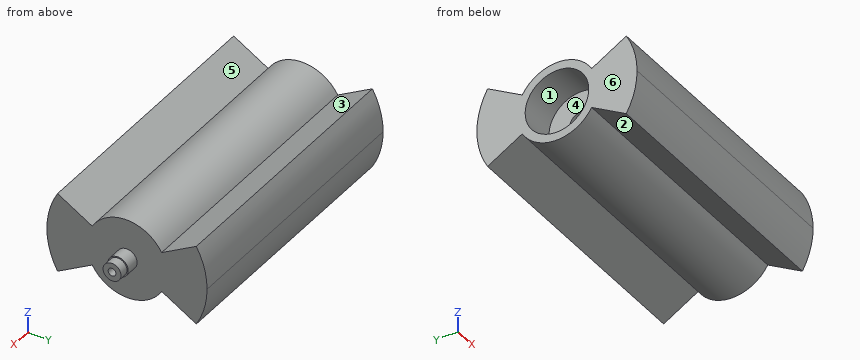
Autodesk Inventor part; units mm, degrees
ref_plane "YZ Plane" through (0, 0, 0) normal (1, 0, 0) x (0, 1, 0)
ref_plane "XZ Plane" through (0, 0, 0) normal (0, 1, 0) x (-1, 0, 0)
ref_plane "XY Plane" through (0, 0, 0) normal (0, 0, 1) x (1, 0, 0)
sketch "Sketch1" plane through (0, 0, 0) normal (1, 0, 0) x (0, 1, 0)
  circle A0 centre (0, 0) radius 17.5
  dimension "d1" = 35
extrude "Extrusion1" add sketch "Sketch1" along normal blind 118
sketch "Sketch2" plane through (0, 0, 0) normal (-1, 0, 0) x (0, 0, 1)
  circle A0 centre (0, 0) radius 13.9
  dimension "d4" = 27.8
extrude "Extrusion2" cut sketch "Sketch2" against normal blind 16
sketch "Sketch3" plane through (16, 0, 0) normal (-1, 0, 0) x (0, 0, 1)
  circle A0 centre (0, 0) radius 4.85
  dimension "d7" = 9.7
extrude "Extrusion3" cut sketch "Sketch3" against normal blind 4.2
sketch "Sketch4" plane through (20.2, 0, 0) normal (-1, 0, 0) x (0, 0, 1)
  circle A0 centre (0, 0) radius 1.7
  dimension "d10" = 3.4
extrude "Extrusion4" cut sketch "Sketch4" against normal blind 10
sketch "Sketch9" plane through (0, 0, 0) normal (1, 0, 0) x (0, 1, 0)
  circle A0 centre (0, 0) radius 1.7 construction
  circle A1 centre (0, 0) radius 35 construction
  line L0 (-35, 0) -> (-17.5, 0)
  circle A2 centre (0, 0) radius 17.5 construction
  line L1 (-15.1554, 8.75) -> (-30.3109, 17.5)
  arc A3 (-30.3109, 17.5) -> (-35, 0) centre (0, 0) ccw
  arc A4 (-15.1554, 8.75) -> (-17.5, 0) centre (0, 0) ccw
  dimension "d32" = 70
  dimension "d33" = 30
extrude "Extrusion8" add sketch "Sketch9" along normal up to surface (118 mm away)
sketch "Sketch10" plane through (118, 0, 0) normal (1, 0, 0) x (0, 0, -1)
  circle A0 centre (0, 0) radius 1.7
  circle A1 centre (0, 0) radius 3.925
  dimension "d36" = 7.85
extrude "Extrusion9" add sketch "Sketch10" along normal blind 10
sketch "Sketch12" plane through (118, 0, 0) normal (1, 0, 0) x (0, 0, -1)
  circle A0 centre (0, 0) radius 4.445
  dimension "d42" = 8.89
extrude "Extrusion11" add sketch "Sketch12" along normal blind 6
sketch "Sketch11" plane through (118, 0, 0) normal (1, 0, 0) x (0, 0, -1)
  circle A0 centre (0, 0) radius 4.85
  circle A1 centre (0, 0) radius 1.7
extrude "Extrusion10" cut sketch "Sketch11" against normal blind 20 from surface at 10 contours A1
mirror "Mirror1" about plane through (0, 0, 0) normal (0, 0, 1) of "Extrusion8"
mirror "Mirror2" about plane through (0, 0, 0) normal (0, 1, 0) of "Extrusion8", "Mirror1"
properties part number "newDrum_3DPrint"
Geometry check sheet. Reference: the model listing, model coordinates, mm. Face numbers are marked on the shaded views. A direction names the side the tool comes from. Round coordinates to 2 decimals unless told otherwise and drop trailing zeros. Write each loop counter-clockwise with the first axis right and the second up, starting at its lowest first coordinate (ties: lowest second). Pieces come first, ordered by that corner, then holes. Notation, with made-up numbers: (-29, -33.75) -> (-8, -33.75) arc R8 ccw to (-8, -29.75) -> close; hole circle Ø3 at (16, 28). An arc over 180 degrees is marked (long way). One line per item, written item: value. Start each with the question number.
(1) Access from +Z, -Z, +X, -X, +Y, -Y to the whole of each face (thin tool, end or side, straight path). Record for the marked faces 1, 2 and 3.
(2) Go/stop test with flat-tipped pins: pin 1 Ø1.5 at (x, z) = (49.5, -9) entering from +Y; pin 2 Ø1.7 at (y, z) = (-0.5, 0) entering from -X; pin 3 Ø8 at (y, z) = (-1, 5.5) entering from -X. Record where each tip stops, or that it passes through.
(3) Scan lines: line 1 (Y direction, x = 23.75, z = 0); line 2 (Y direction, x = 19, z = 0); line 3 (Y direction, x = 107, z = -16). Record each from-to range of solid material in increasing order. Write a range as [from, to].
(4) Cross-section at C-C, the plane x = 47. Record the cut outline in (y, z), and give its area (3 significant figures).
(5) Cross-section at B-B, the plane y = 0. Record the cut outline in (x, z) (3 decimals), and give its area (3 significant figures).
(6) Draft check along Z on the marked faces 4, 5 and 6. Enter one of: +Z half, -Z half, draft (parallel to the pull), parting line (faces both ways), or undercut.
(7) Cross-section at D-D, the plane z = -7. Record the cut outline in (x, y), and give its area (3 significant figures).
(8) Cross-section at A-A, the plane x = 13. Record the cut outline in (y, z), and give its area (3 significant figures).
Answer:
1. face 1: -X
1. face 2: -Z, +X, -X
1. face 3: +Z, +X, -X
2. pin 1: y = 34.01
2. pin 2: x = 30.2
2. pin 3: x = 16
3. line 1: [-35, -1.7], [1.7, 35]
3. line 2: [-35, -4.85], [4.85, 35]
3. line 3: [-31.13, -27.71], [-7.09, 7.09], [27.71, 31.13]
4. outline: (-35, 0) arc R35 ccw to (-30.31, -17.5) -> (-15.16, -8.75) arc R17.5 ccw to (15.16, -8.75) -> (30.31, -17.5) arc R35 ccw to (35, 0) arc R35 ccw to (30.31, 17.5) -> (15.16, 8.75) arc R17.5 ccw to (-15.16, 8.75) -> (-30.31, 17.5) arc R35 ccw to start
4. area: 1,920 mm²
5. outline: (0, -17.5) -> (118, -17.5) -> (118, -4.445) -> (124, -4.445) -> (124, -3.925) -> (128, -3.925) -> (128, -1.7) -> (108, -1.7) -> (108, 1.7) -> (128, 1.7) -> (128, 3.925) -> (124, 3.925) -> (124, 4.445) -> (118, 4.445) -> (118, 17.5) -> (0, 17.5) -> (0, 13.9) -> (16, 13.9) -> (16, 4.85) -> (20.2, 4.85) -> (20.2, 1.7) -> (30.2, 1.7) -> (30.2, -1.7) -> (20.2, -1.7) -> (20.2, -4.85) -> (16, -4.85) -> (16, -13.9) -> (0, -13.9) -> close
5. area: 3,630 mm²
6. face 4: undercut
6. face 5: +Z half
6. face 6: draft
7. outline: (0, -34.29) -> (118, -34.29) -> (118, 34.29) -> (0, 34.29) -> (0, 12.01) -> (16, 12.01) -> (16, -12.01) -> (0, -12.01) -> close
7. area: 7,710 mm²
8. outline: (-35, 0) arc R35 ccw to (-30.31, -17.5) -> (-15.16, -8.75) arc R17.5 ccw to (15.16, -8.75) -> (30.31, -17.5) arc R35 ccw to (35, 0) arc R35 ccw to (30.31, 17.5) -> (15.16, 8.75) arc R17.5 ccw to (-15.16, 8.75) -> (-30.31, 17.5) arc R35 ccw to start; hole circle Ø27.8 at (0, 0)
8. area: 1,320 mm²
